from build123d import *

# Parameters (mm, degrees)
SKETCH1_W           = 25.4
SKETCH1_H           = 19.05
BOSS_EXTRUDE1_DEPTH = 12.7
SKETCH2_R           = 4.7625
CUT_EXTRUDE1_DEPTH  = 35.195796525
FILLET1_R           = 3.175


with BuildPart() as part:
    # Sketch1 → Boss-Extrude1 (new body)
    with BuildSketch(Plane(origin=(0, 0, 0), x_dir=(1, 0, 0), z_dir=(0, 1, 0))):
        with Locations((12.7, 9.525)):
            Rectangle(SKETCH1_W, SKETCH1_H)
    extrude(amount=BOSS_EXTRUDE1_DEPTH)

    # Sketch2 → Cut-Extrude1 (cut, through all)
    with BuildSketch(Plane(origin=(0, 12.7, 0), x_dir=(1, 0, 0), z_dir=(0, 1, 0))):
        with Locations(Location((12.7, 9.525, 0), (0, 0, 270))):
            Circle(SKETCH2_R)
    extrude(amount=-CUT_EXTRUDE1_DEPTH, mode=Mode.SUBTRACT)

    # Fillet1
    fillet1_edges = [part.edges().sort_by_distance(p)[0] for p in [
        (0, 6.35, -19.05),
        (25.4, 6.35, -19.05),
    ]]
    fillet(fillet1_edges, radius=FILLET1_R)


solid = part.part
For this review, take the finished solid that the model builds, in its own axes (mm). Round coordinates to 2 decimals unless told otherwise and drop trailing zeros. Loops run counter-clockwise (first coordinate to the right, second up) from the corner with the lowest first, then second, coordinate; pieces in that order, holes last. Notation, with made-up numbers: (-7, -15) - (9, -15) arc R24 cw to (9, 5) - close; hole circle Ø4 at (78.25, 38.25). An arc over 180 degrees is marked (long way). One line per item, written item: value. Start each with the question number.
Item 1: Take a section at B-B (x = 12.7). Give the boundary of the cut face in (y, z), plus the area to 3 significant figures.
Item 2: Take a section at C-C (z = -11). Give the boundary of the cut face in (x, y).
Item 3: For L1, parallel to Z at x = 12.5, y = 3.75; L2, parallel to X at y = 4.5, z = -6.75; L3, parallel to Z at x = 10, y = 6, list the stretches that pass through material, from the lowest coordinate up.
Answer below:
1. outline: (0, -19.05) - (12.7, -19.05) - (12.7, -14.29) - (0, -14.29) - close; (0, -4.76) - (12.7, -4.76) - (12.7, 0) - (0, 0) - close
1. area: 121 mm2
2. outline: (0, 0) - (8.17, 0) - (8.17, 12.7) - (0, 12.7) - close; (17.23, 0) - (25.4, 0) - (25.4, 12.7) - (17.23, 12.7) - close
3. L1: z = -19.05 to -14.28, -4.77 to 0
3. L2: x = 0 to 8.83, 16.57 to 25.4
3. L3: z = -19.05 to -13.45, -5.6 to 0
